from build123d import *

# Parameters (mm, degrees)
SALIENTE_EXTRUIR1_DEPTH = 47.5
SALIENTE_EXTRUIR2_DEPTH = 51.556282
SALIENTE_EXTRUIR3_DEPTH = 51.556282


with BuildPart() as part:
    # Croquis1 → Saliente-Extruir1 (new, symmetric)
    with BuildSketch(Plane.XY):
        Polygon((44.649051179, 25.778141718), (0, 51.556283435), (-44.649051179, 25.778141718), (-44.649051179, -25.778141718), (0, -51.556283435), (44.649051179, -25.778141718), align=None)
    extrude(amount=SALIENTE_EXTRUIR1_DEPTH, both=True)

    # Croquis6 → Saliente-Extruir2 (add)
    with BuildSketch(Plane(origin=(22.32452559, 12.889070859, 0), x_dir=(0, 0, -1), z_dir=(-0.8660254037844388, -0.49999999999999983, 0))):
        with BuildLine():
            Line((-47.516964524, 44.649051179), (47.5, 44.649051179))
            Line((47.5, 44.649051179), (47.5, 125.450551246))
            add(Edge.make_bspline(
                [(47.5, 125.450551246), (28.48813233, 69.96313115), (-47.516964524, 44.649051179)],
                knots=[0, 0, 0, 1, 1, 1], degree=2))
        make_face()
    extrude(amount=SALIENTE_EXTRUIR2_DEPTH)

    # Croquis8 → Saliente-Extruir3 (add)
    with BuildSketch(Plane(origin=(0, 25.778141718, 0), x_dir=(0, 0, -1), z_dir=(0, 1, 0))):
        with BuildLine():
            Line((47.5, 44.649051179), (47.5, 125.452857029))
            add(Edge.make_bspline(
                [(47.5, 125.452857029), (28.489618358, 69.977349558), (-47.490800068, 44.66905118)],
                knots=[0, 0, 0, 1, 1, 1], degree=2))
            Line((-47.490800068, 44.66905118), (-47.5, 44.649051179))
            Line((-47.5, 44.649051179), (47.5, 44.649051179))
        make_face()
    extrude(amount=-SALIENTE_EXTRUIR3_DEPTH)


solid = part.part
Here's how the part is built. I have some questions about the finished solid (model axes, mm). A direction names the side the tool comes from. Round coordinates to 2 decimals unless told otherwise and drop trailing zeros. Order: outer loops, then holes, each group sorted by start corner. A loop starts at its lowest first (then second) coordinate and runs counter-clockwise, first axis right, second up. Notation, with made-up numbers: (46.25, 68) -> (61.25, 68) arc R10 cw to (61.25, 87) -> close; hole circle Ø5 at (-24.5, 48.5). An arc over 180 degrees is marked (long way). Use CSV: the item, a comma, the result in double quotes.
1. I want a section at B-B on y = 41. List the corners of the cut face in (x, z) for me.
Recorded:
outline,"(-18.28, -47.5) -> (18.28, -47.5) -> (18.28, 47.5) -> (-18.28, 47.5) -> close"
2. I'm going to push flat-ended pins straight in: P1, Ø24, axis at x = -72.5, z = -13, coming from the -Y side; P2, Ø6, axis at y = 16, z = 27.5, coming from the -X side; P3, Ø2, axis at x = 17.5, y = -68.5, coming from the +Z side; P4, Ø24, axis at x = -77, z = 10, coming from the +Y side. Where does each tip first touch, or does it pass through?
Recorded:
P1,"stops at y = -25.78"
P2,"stops at x = -53.6"
P3,"stops at z = -0.26"
P4,"passes through"
3. Which directions (+Z, -Z, +X, -X, +Y, -Y) give clear straight access to the entire face, cutting with the end or side of a thin tool? Please do faces 1 (the face through (-1, 1, 47.5)), 2 (the face through (-67, 25.778, -17)), 3 (the face through (-19, -15, -47.5)), 4 (the face through (44.649, 0, 1)), 5 (the face through (-67, -25.778, -17)).
Recorded:
face 1,"+Z, +X, -X, +Y, -Y"
face 2,"+Z, -Z, -X, +Y"
face 3,"-Z, +X, -X, +Y, -Y"
face 4,"+Z, -Z, +X, +Y"
face 5,"+Z, -Z, -X, -Y"
4. I want a section at A-A on x = -14.5. List the corners of the cut face in (y, z) for me, and give its area (3 significant figures).
Recorded:
outline,"(-43.18, -47.5) -> (43.18, -47.5) -> (43.18, 47.5) -> (-43.18, 47.5) -> close"
area,"8,210 mm2"
5. I need wall thicknesses on line 1 along X through (y, z) = (-20, 39.5); line 2 along Z through (x, y) = (7, -40); line 3 along Y through (x, z) = (24.5, 22). Which ranges of each line are inside material? Lowest first, please.
Recorded:
line 1,"x = -47.47 to 44.65"
line 2,"z = -47.5 to 47.5"
line 3,"y = -49.06 to 37.41"
